from build123d import *
from build123d.topology import SkipClean

# Parameters (mm, degrees)
BOSS_EXTRUDE1_DEPTH = 7.87
SKETCH2_R           = 2.45
BOSS_EXTRUDE2_DEPTH = 1.8
SKETCH3_R           = 2.45
SKETCH3_R_2         = 1.57
BOSS_EXTRUDE3_DEPTH = 1.77
SKETCH4_R           = 1.57
CUT_EXTRUDE1_DEPTH  = 16.324578298
SKETCH5_W           = 4.87
SKETCH5_H           = 4.81
CUT_EXTRUDE2_DEPTH  = 4.92
SKETCH6_W           = 4.97
SKETCH6_H           = 4.9
CUT_EXTRUDE3_DEPTH  = 8.81
SHELL1_START        = 8.81
SHELL1_OUTLINE_R    = 0.95
SHELL1_DEPTH        = 1.16


# Read off the part's stored shape, not the designer's step: Shell1
with BuildPart() as part:
    # Sketch1 → Boss-Extrude1 (new body)
    with BuildSketch(Plane(origin=(0, 0, 0), x_dir=(0, 0, -1), z_dir=(1, 0, 0))):
        Polygon((0, 0), (0, 9.67), (-6.43, 9.67), (-6.43, 1.61), (-7.9, 1.61), (-7.9, 0), align=None)
    extrude(amount=-BOSS_EXTRUDE1_DEPTH)

    # Sketch2 → Boss-Extrude2 (add)
    with BuildSketch(Plane(origin=(0, 9.67, 0), x_dir=(1, 0, 0), z_dir=(0, 1, 0))):
        with Locations(Location((-3.935, -3.95, 0), (0, 0, 270))):
            Circle(SKETCH2_R)
    extrude(amount=BOSS_EXTRUDE2_DEPTH)

    # Sketch3 → Boss-Extrude3 (add)
    with BuildSketch(Plane.XY.offset(6.43)):
        with Locations((-3.935, 5.65)):
            Circle(SKETCH3_R)
        with Locations(Location((-3.935, 5.65, 0), (0, 0, 270))):
            Circle(SKETCH3_R_2, mode=Mode.SUBTRACT)
    extrude(amount=BOSS_EXTRUDE3_DEPTH)

    # Sketch4 → Cut-Extrude1 (cut, through all)
    with SkipClean():  # the faces are left unmerged after this step: merging them gives an invalid solid
        with BuildSketch(Plane.XY.offset(6.43)):
            with Locations((-3.935, 5.65)):
                Circle(SKETCH4_R)
        extrude(amount=-CUT_EXTRUDE1_DEPTH, mode=Mode.SUBTRACT)

    # Sketch5 → Cut-Extrude2 (cut)
    with SkipClean():  # the faces are left unmerged after this step: merging them gives an invalid solid
        with BuildSketch(Plane(origin=(0, 0, 0), x_dir=(-1, 0, 0), z_dir=(0, 0, -1))):
            with Locations((3.935, 5.705)):
                Rectangle(SKETCH5_W, SKETCH5_H)
        extrude(amount=-CUT_EXTRUDE2_DEPTH, mode=Mode.SUBTRACT)

    # Sketch6 → Cut-Extrude3 (cut)
    with SkipClean():  # the faces are left unmerged after this step: merging them gives an invalid solid
        with BuildSketch(Plane.XZ):
            with Locations((-3.935, 3.95)):
                Rectangle(SKETCH6_W, SKETCH6_H)
        extrude(amount=-CUT_EXTRUDE3_DEPTH, mode=Mode.SUBTRACT)

    # Shell1 outline → Shell1 (cut)
    with SkipClean():  # the faces are left unmerged after this step: merging them gives an invalid solid
        with BuildSketch(Plane(origin=(0, 0, 0), x_dir=(1, 0, 0), z_dir=(0, 1, 0)).offset(SHELL1_START)):
            with Locations((-3.935, -3.95)):
                Circle(SHELL1_OUTLINE_R)
        extrude(amount=SHELL1_DEPTH, mode=Mode.SUBTRACT)


solid = part.part
Could you check a few things on this model? Use its own coordinates, in mm. A direction names the side the tool comes from. Give positions to 0.01 mm unless a question says otherwise; leave off trailing zeros. Order: outer loops, then holes, each group sorted by start corner. A loop starts at its lowest first (then second) coordinate and runs counter-clockwise, first axis right, second up. Notation, with made-up numbers: (7, 61.25) -> (11, 61.25) arc R11 cw to (11, 67.25) -> close; hole circle Ø10 at (32, 68.5). An arc over 180 degrees is marked (long way). Return JSON: item names as keys, results as strings.
1. Imagine slicing it at B-B on x = -2.5. List the corners of the cut face in (y, z) for me.
Answer list:
{"outline": "(0, 0) -> (3.3, 0) -> (3.3, 1.5) -> (0, 1.5) -> close; (0, 6.4) -> (5.01, 6.4) -> (5.01, 8.2) -> (3.66, 8.2) -> (3.66, 6.43) -> (1.61, 6.43) -> (1.61, 7.9) -> (0, 7.9) -> close; (6.29, 6.4) -> (8.81, 6.4) -> (8.81, 1.5) -> (8.11, 1.5) -> (8.11, 0) -> (9.67, 0) -> (9.67, 1.96) -> (11.47, 1.96) -> (11.47, 5.94) -> (9.67, 5.94) -> (9.67, 6.43) -> (7.64, 6.43) -> (7.64, 8.2) -> (6.29, 8.2) -> close"}
2. Imagine slicing it at A-A on y = 9.5. List the corners of the cut face in (x, z) for me (3 decimals).
Answer list:
{"outline": "(-7.87, 0) -> (0, 0) -> (0, 6.43) -> (-7.87, 6.43) -> close; hole circle Ø1.9 at (-3.935, 3.95)"}
3. Imagine slicing it at D-D on z = 3.95. List the corners of the cut face in (x, y) for me (3 decimals).
Answer list:
{"outline": "(-7.87, 0) -> (-6.42, 0) -> (-6.42, 8.81) -> (-4.885, 8.81) -> (-4.885, 9.97) -> (-2.985, 9.97) -> (-2.985, 8.81) -> (-1.45, 8.81) -> (-1.45, 0) -> (0, 0) -> (0, 9.67) -> (-1.485, 9.67) -> (-1.485, 11.47) -> (-6.385, 11.47) -> (-6.385, 9.67) -> (-7.87, 9.67) -> close"}
4. On a 3-axis mill with a long thin cutter (end or side, diameter ignored), from which of +Z, -Z, +X, -X, +Y, -Y can I reach the whole of each face in a straight line? I mean faces 1 (the flat face through (-4, 8.11, 1)), 2 (the flat face through (-1, 6, 6.43)), 3 (the flat face through (-4, 1, 7.9)), 4 (the flat face through (-1.45, 4, 4)). Say none if no direction works.
Answer list:
{"face 1": "-Z", "face 2": "+Z", "face 3": "+Z, +X, -X, -Y", "face 4": "-Y"}
5. Thinking about a two-plate mould opening in Z: for faces 5 (the flat face through (-7.87, 5, 3)), 6 (the flat face through (-4, 2, 1.5)), 7 (the cylindrical face through (-3.199, 10.557, 6.287)), which applies, pulls with the +Z half, pulls with the -Z half, needs draft (parallel to the pull), parting line crosses it, or undercut?
Answer list:
{"face 5": "needs draft", "face 6": "undercut", "face 7": "parting line crosses it"}
6. I need wall thicknesses on line 1 (Y direction, x = -5, z = 6.5); line 2 (X direction, y = 2.5, z = 3.75); line 3 (Z direction, x = -4.5, y = 1.5). Which ranges of each line are inside material? Lowest first, please. Write a range as from..to.
Answer list:
{"line 1": "y = 0..1.61, 3.44..4.5, 6.8..7.86", "line 2": "x = -7.87..-6.42, -1.45..0", "line 3": "z = 0..1.5, 6.4..7.9"}
7. Imagine slicing it at C-C on y = 5.65. List the corners of the cut face in (x, z) for me (3 decimals), then the cut area to 3 significant figures.
Answer list:
{"outline": "(-7.87, 0) -> (-6.37, 0) -> (-6.37, 1.5) -> (-6.42, 1.5) -> (-6.42, 6.4) -> (-5.505, 6.4) -> (-5.505, 8.2) -> (-6.385, 8.2) -> (-6.385, 6.43) -> (-7.87, 6.43) -> close; (-2.365, 6.4) -> (-1.45, 6.4) -> (-1.45, 1.5) -> (-1.5, 1.5) -> (-1.5, 0) -> (0, 0) -> (0, 6.43) -> (-1.485, 6.43) -> (-1.485, 8.2) -> (-2.365, 8.2) -> close", "area": "22.0 mm2"}
8. For pin 1 Ø2.5 at (x, y) = (-3.935, 5.65) entering from +Z; pin 2 Ø0.9 at (x, z) = (-3.5, 3.5) entering from -Y; pin 3 Ø0.7 at (x, z) = (-6, 7) entering from +Y; pin 4 Ø0.5 at (x, y) = (-3.5, 1) entering from +Z, each with a flat end and sliding along its axis, tell me the tip position at first contact or that it passes through.
Answer list:
{"pin 1": "passes through", "pin 2": "stops at y = 8.81", "pin 3": "stops at y = 7.4", "pin 4": "stops at z = 7.9"}
